Verification items for this drawing (mm, ordinates from the low corner). Round coordinates to 2 decimals unless told otherwise and drop trailing zeros. Loops run counter-clockwise (first coordinate to the right, second up) from the corner with the lowest first, then second, coordinate; pieces in that order, holes last. Notation, with made-up numbers: (-33, 38.25) -> (-28, 38.25) arc R21 ccw to (-28, 43.25) -> close; hole circle Ø11 at (-31.5, -7). An arc over 180 degrees is marked (long way). One line per question, with ' | ' between items.
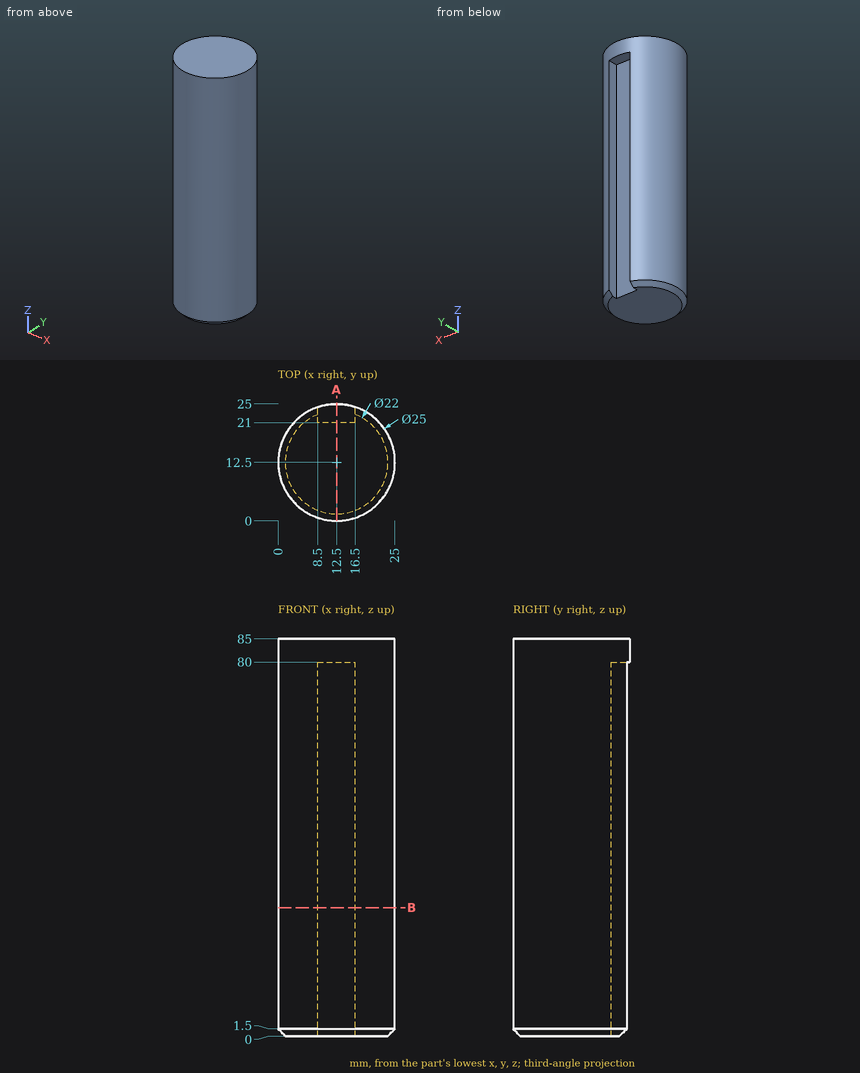
(1) Go/stop test with flat-tipped pins: pin 1 (4.5 mm diameter, centred on x = 13, y = 24, fed in from -Z); pin 2 (9 mm diameter, centred on x = 14.5, z = 39, fed in from +Y); pin 3 (1.5 mm diameter, centred on y = 10.5, z = 67, fed in from -X). Record where each tip stops, or that it passes through.
Answer:
pin 1: stops at z = 80 | pin 2: stops at y = 24.34 | pin 3: stops at x = 0.06
(2) Sectioned sample at B-B, the plane z = 27.5. Record the cut outline in (x, y), and give its area (3 significant figures).
Answer:
outline: (8.5, 21) -> (8.5, 24.34) arc R12.5 ccw (long way) to (16.5, 24.34) -> (16.5, 21) -> close | area: 461 mm2
(3) Sectioned sample at A-A, the plane x = 12.5. Record the cut outline in (y, z), and give its area (3 significant figures).
Answer:
outline: (0, 1.5) -> (1.5, 0) -> (21, 0) -> (21, 80) -> (25, 80) -> (25, 85) -> (0, 85) -> close | area: 1,800 mm2
(4) Scan lines: probe 1 along X at (y, z) = (12.75, 35); probe 2 along X at (y, z) = (23, 36); probe 3 along Z at (x, y) = (15, 21.75). Record each from-to range of solid material in increasing order.
Answer:
probe 1: x = 0 to 25 | probe 2: x = 5.72 to 8.5, 16.5 to 19.28 | probe 3: z = 80 to 85
